Work out the finished part from the listing and answer in its coordinate system (mm). Face numbers are marked on the shaded views. A direction names the side the tool comes from. Coordinates: 2 decimals unless noted, no trailing zeros. Loops run counter-clockwise (first coordinate to the right, second up) from the corner with the lowest first, then second, coordinate; pieces in that order, holes last. Notation, with made-up numbers: (76, 2) - (129, 2) arc R21 cw to (129, 36) - close; hole circle Ø10 at (16, -5). An arc over 180 degrees is marked (long way). Write each question's results on one line, items separated by ' | '. Start each with the question number.
Item 1: Section A-A, the plane y = 10.5 is taken. Write down the section's boundary in (x, z), plus the area to 3 significant figures.
Item 2: Consider probe 1 along Y at (x, z) = (6, 1.1); probe 2 along X at (y, z) = (10.5, 1.2); probe 3 along X at (y, z) = (30.5, 0.85). Determine where each line is inside the solid, lowest interval first. Write a range as [from, to].
Item 3: Section B-B, the plane x = 6 is taken. Write down the section's boundary in (y, z).
Item 4: A tool of negligible diameter and unlimited length cuts with its end or side. For the marked faces 3 and 4, from which of +Z, -Z, +X, -X, +Y, -Y can it reach the whole face along a straight path? Write none if from no direction.
Item 5: Section C-C, the plane x = 17.5 is taken. Write down the section's boundary in (y, z).
Item 6: Each of these flat-tipped pins is pushed along its axis until it touches: pin 1 Ø0.8 at (x, z) = (-16.5, 1.5) entering from +Y; pin 2 Ø2.5 at (x, y) = (35.64, 77.25) entering from -Z; pin 3 Ø8 at (x, y) = (11, 54.5) entering from +Z. Where does it stop, or does it pass through?
Item 7: Section D-D, the plane y = 114.6 is taken. Write down the section's boundary in (x, z), plus the area to 3 significant figures.
Item 8: For a pull along Y with two mould halves and no side action, classify the marked faces 1 and 2 as +Y half, -Y half, draft (parallel to the pull), parting line (faces both ways), or undercut.
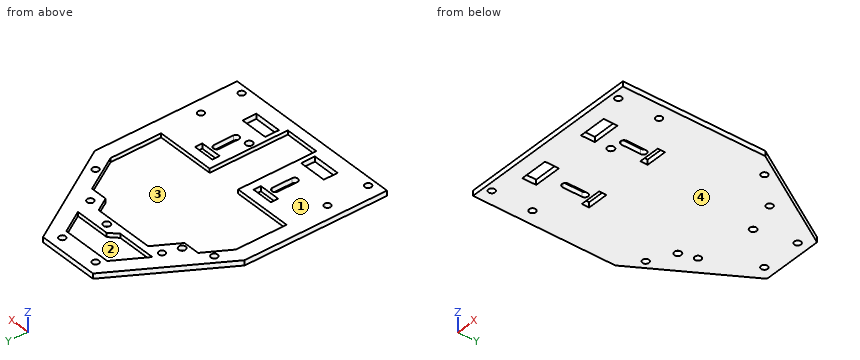
from build123d import *

# Parameters (mm, degrees)
PAD_DEPTH       = 2.5
SKETCH001_R     = 1.6
SKETCH001_W     = 13.6
SKETCH001_H     = 6.8
SKETCH001_W_2   = 10.4
SKETCH001_H_2   = 3.6
POCKET_DEPTH    = 5
SKETCH002_R     = 1.7
POCKET001_DEPTH = 5
SKETCH004_R     = 1.6
POCKET002_DEPTH = 5
POCKET003_DEPTH = 2


with BuildPart() as part:
    # Sketch → Pad (new body)
    with BuildSketch(Plane.XY):
        Polygon((-45, 0), (45, 0), (45, 70), (15, 120), (-15, 120), (-45, 70), align=None)
    extrude(amount=PAD_DEPTH)

    # Sketch001 (on Face8 of Pad) → Pocket (cut)
    with BuildSketch(Plane.XY.offset(2.5)):
        with Locations((38, 3.5)):
            Circle(SKETCH001_R)
        with Locations((38, 23.5)):
            Circle(SKETCH001_R)
        with Locations((-38, 3.5)):
            Circle(SKETCH001_R)
        with Locations((-38, 23.5)):
            Circle(SKETCH001_R)
        with BuildLine():
            ThreePointArc((-19.2, 23), (-17.6, 21.4), (-16, 23))
            Line((-16, 23), (-16, 32.5))
            ThreePointArc((-16, 32.5), (-17.6, 34.1), (-19.2, 32.5))
            Line((-19.2, 23), (-19.2, 32.5))
        make_face()
        with BuildLine():
            ThreePointArc((19.2, 32.5), (17.6, 34.1), (16, 32.5))
            Line((16, 32.5), (16, 23))
            ThreePointArc((16, 23), (17.6, 21.4), (19.2, 23))
            Line((19.2, 32.5), (19.2, 23))
        make_face()
        with Locations((-17.6, 10.8)):
            Rectangle(SKETCH001_W, SKETCH001_H)
        with Locations((17.6, 10.8)):
            Rectangle(SKETCH001_W, SKETCH001_H)
        with Locations((17.6, 37.1)):
            Rectangle(SKETCH001_W_2, SKETCH001_H_2)
        with Locations((-17.6, 37.1)):
            Rectangle(SKETCH001_W_2, SKETCH001_H_2)
    extrude(amount=-POCKET_DEPTH, mode=Mode.SUBTRACT)

    # Sketch002 (on Face5 of Pocket) → Pocket001 (cut)
    with BuildSketch(Plane.XY.offset(2.5)):
        with Locations((6, 96)):
            Circle(SKETCH002_R)
        with Locations((-24, 83.5)):
            Circle(SKETCH002_R)
        with Locations((11.5, 21.5)):
            Circle(SKETCH002_R)
    extrude(amount=-POCKET001_DEPTH, mode=Mode.SUBTRACT)

    # Sketch004 (on Face5 of Pocket001) → Pocket002 (cut)
    with BuildSketch(Plane.XY.offset(2.5)):
        with Locations((10, 114.6)):
            Circle(SKETCH004_R)
        with Locations((-10, 114.6)):
            Circle(SKETCH004_R)
        with Locations((21.5, 91.3880009298)):
            Circle(SKETCH004_R)
        with Locations((35.6421356237, 77.2458653061)):
            Circle(SKETCH004_R)
        with Locations((-21.5, 91.3880009298)):
            Circle(SKETCH004_R)
        with Locations((-35.6421356237, 77.2458653061)):
            Circle(SKETCH004_R)
    extrude(amount=-POCKET002_DEPTH, mode=Mode.SUBTRACT)

    # Sketch003 (on Face5 of Pocket002) → Pocket003 (cut)
    with BuildSketch(Plane.XY.offset(2.5)):
        Polygon((-37.6466903558, 43.3474069665), (-8.5768340117, 43.3474069665), (-8.5768340117, 4.893821), (8.5768340117, 4.893821), (8.5768340117, 43.3474069665), (37.6466903558, 43.3474069665), (37.6466903558, 68.2449686275), (27.0264066989, 86.0525109264), (18.8520822966, 86.0525109264), (14.8551351559, 92.7543851488), (-14.8551351559, 92.7543851488), (-22.0103766194, 80.7568463697), (-30.1847010216, 80.7568463697), (-37.6466903558, 68.2449686275), align=None)
        Polygon((-21.162924581, 95.8840944515), (-1.9676886795, 95.8840944515), (1.694907, 99.5545331507), (18.973902678, 99.5545331507), (12.2977542374, 110.7487535303), (-12.2977542374, 110.7487535303), align=None)
    extrude(amount=-POCKET003_DEPTH, mode=Mode.SUBTRACT)


solid = part.part
Answer key:
1) outline: (-45, 0) - (-24.4, 0) - (-24.4, 2.5) - (-45, 2.5) - close; (-10.8, 0) - (10.8, 0) - (10.8, 2.5) - (8.58, 2.5) - (8.58, 0.5) - (-8.58, 0.5) - (-8.58, 2.5) - (-10.8, 2.5) - close; (24.4, 0) - (45, 0) - (45, 2.5) - (24.4, 2.5) - close | area: 123 mm^2
2) probe 1: y = [0, 4.89], [92.75, 94.3], [97.7, 99.55], [110.75, 120] | probe 2: x = [-45, -24.4], [-10.8, -8.58], [8.58, 10.8], [24.4, 45] | probe 3: x = [-45, -19.2], [-16, -8.58], [8.58, 16], [19.2, 45]
3) outline: (0, 0) - (94.3, 0) - (94.3, 2.5) - (92.75, 2.5) - (92.75, 0.5) - (4.89, 0.5) - (4.89, 2.5) - (0, 2.5) - close; (97.7, 0) - (120, 0) - (120, 2.5) - (110.75, 2.5) - (110.75, 0.5) - (99.55, 0.5) - (99.55, 2.5) - (97.7, 2.5) - close
4) face 3: +Z | face 4: -Z, +X, -X, +Y, -Y
5) outline: (0, 0) - (7.4, 0) - (7.4, 2.5) - (0, 2.5) - close; (14.2, 0) - (21.4, 0) - (21.4, 2.5) - (14.2, 2.5) - close; (34.1, 0) - (35.3, 0) - (35.3, 2.5) - (34.1, 2.5) - close; (38.9, 0) - (115.83, 0) - (115.83, 2.5) - (102.03, 2.5) - (102.03, 0.5) - (99.55, 0.5) - (99.55, 2.5) - (88.32, 2.5) - (88.32, 0.5) - (43.35, 0.5) - (43.35, 2.5) - (38.9, 2.5) - close
6) pin 1: stops at y = 118.17 | pin 2: passes through | pin 3: stops at z = 0.5
7) outline: (-18.24, 0) - (-11.6, 0) - (-11.6, 2.5) - (-18.24, 2.5) - close; (-8.4, 0) - (8.4, 0) - (8.4, 2.5) - (-8.4, 2.5) - close; (11.6, 0) - (18.24, 0) - (18.24, 2.5) - (11.6, 2.5) - close | area: 75.2 mm^2
8) face 1: draft | face 2: undercut
